```python
from build123d import *

# Parameters (mm, degrees)
SKETCH1_R           = 3.175
BOSS_EXTRUDE1_DEPTH = 2.794
SKETCH2_R           = 11.049
SKETCH2_R_2         = 15.875
SKETCH2_R_3         = 1.27
CUT_EXTRUDE1_DEPTH  = 202.908472752
ITC_CUTOUT_DEPTH    = 202.908472752
SKETCH6_W           = 67.523241089
SKETCH6_H           = 6.35
CUT_EXTRUDE3_DEPTH  = 202.908472752
FILLET1_R           = 6.35
CUT_EXTRUDE4_DEPTH  = 202.908472752
FILLET2_R           = 6.35
SKETCH8_R           = 1.5875
CUT_EXTRUDE5_DEPTH  = 202.908472752
SKETCH10_R          = 1.5875
CUT_EXTRUDE6_DEPTH  = 202.908472752
SKETCH11_R          = 1.5875
CUT_EXTRUDE7_DEPTH  = 202.908472752


with BuildPart() as part:
    # Sketch1 → Boss-Extrude1 (new, symmetric)
    with BuildSketch(Plane.XY):
        with BuildLine():
            Line((-145.783553311, 66.675), (145.783553311, 66.675))
            ThreePointArc((145.783553311, 66.675), (147.900219978, 66.497368874), (149.957676269, 65.969444444))
            ThreePointArc((149.957676269, 65.969444444), (172.789871953, 52.74760778), (189.088888889, 31.999880883))
            ThreePointArc((189.088888889, 31.999880883), (190.142181511, 29.17513943), (190.5, 26.181720723))
            Line((190.5, 26.181720723), (190.5, -22.225))
            ThreePointArc((190.5, -22.225), (186.780256121, -31.205256121), (177.8, -34.925))
            Line((177.8, -34.925), (-177.8, -34.925))
            ThreePointArc((-177.8, -34.925), (-186.780256121, -31.205256121), (-190.5, -22.225))
            Line((-190.5, -22.225), (-190.5, 26.181720723))
            ThreePointArc((-190.5, 26.181720723), (-190.142181511, 29.17513943), (-189.088888889, 31.999880883))
            ThreePointArc((-189.088888889, 31.999880883), (-172.789871953, 52.74760778), (-149.957676269, 65.969444444))
            ThreePointArc((-149.957676269, 65.969444444), (-147.900219978, 66.497368874), (-145.783553311, 66.675))
        make_face()
        with Locations((-127, 0)):
            Circle(SKETCH1_R, mode=Mode.SUBTRACT)
        with Locations((127, 0)):
            Circle(SKETCH1_R, mode=Mode.SUBTRACT)
    extrude(amount=BOSS_EXTRUDE1_DEPTH, both=True)

    # Sketch2 → Cut-Extrude1 (cut, through all)
    with BuildSketch(Plane.XY.offset(2.794)):
        with Locations((-127, 0)):
            Circle(SKETCH2_R)
        with Locations((-160.3375, 0)):
            Circle(SKETCH2_R_2)
        with Locations((-143.499519773, 16.837980227)):
            Circle(SKETCH2_R_3)
        with Locations((-160.3375, 23.8125)):
            Circle(SKETCH2_R_3)
        with Locations((-143.499519773, -16.837980227)):
            Circle(SKETCH2_R_3)
        with Locations((-160.3375, -23.8125)):
            Circle(SKETCH2_R_3)
        with Locations((-177.175480227, -16.837980227)):
            Circle(SKETCH2_R_3)
        with Locations((-184.15, 0)):
            Circle(SKETCH2_R_3)
        with Locations((-177.175480227, 16.837980227)):
            Circle(SKETCH2_R_3)
        with Locations((-127, 15.875)):
            Circle(SKETCH2_R_3)
        with Locations((-115.774679849, 11.225320151)):
            Circle(SKETCH2_R_3)
        with Locations((-111.125, 0)):
            Circle(SKETCH2_R_3)
        with Locations((-115.774679849, -11.225320151)):
            Circle(SKETCH2_R_3)
        with Locations((-127, -15.875)):
            Circle(SKETCH2_R_3)
        with Locations((-138.225320151, -11.225320151)):
            Circle(SKETCH2_R_3)
        with Locations(Location((138.225320151, 11.225320151, 0), (0, 0, 180))):
            Circle(SKETCH2_R_3)
        with Locations((-138.225320151, 11.225320151)):
            Circle(SKETCH2_R_3)
        with Locations(Location((138.225320151, -11.225320151, 0), (0, 0, 180))):
            Circle(SKETCH2_R_3)
        with Locations(Location((127, -15.875, 0), (0, 0, 180))):
            Circle(SKETCH2_R_3)
        with Locations(Location((115.774679849, -11.225320151, 0), (0, 0, 180))):
            Circle(SKETCH2_R_3)
        with Locations(Location((111.125, 0, 0), (0, 0, 180))):
            Circle(SKETCH2_R_3)
        with Locations(Location((115.774679849, 11.225320151, 0), (0, 0, 180))):
            Circle(SKETCH2_R_3)
        with Locations(Location((127, 15.875, 0), (0, 0, 180))):
            Circle(SKETCH2_R_3)
        with Locations(Location((177.175480227, 16.837980227, 0), (0, 0, 180))):
            Circle(SKETCH2_R_3)
        with Locations(Location((184.15, 0, 0), (0, 0, 180))):
            Circle(SKETCH2_R_3)
        with Locations(Location((177.175480227, -16.837980227, 0), (0, 0, 180))):
            Circle(SKETCH2_R_3)
        with Locations(Location((160.3375, -23.8125, 0), (0, 0, 180))):
            Circle(SKETCH2_R_3)
        with Locations(Location((143.499519773, -16.837980227, 0), (0, 0, 180))):
            Circle(SKETCH2_R_3)
        with Locations(Location((160.3375, 23.8125, 0), (0, 0, 180))):
            Circle(SKETCH2_R_3)
        with Locations(Location((143.499519773, 16.837980227, 0), (0, 0, 180))):
            Circle(SKETCH2_R_3)
        with Locations(Location((160.3375, 0, 0), (0, 0, 180))):
            Circle(SKETCH2_R_2)
        with Locations(Location((127, 0, 0), (0, 0, 180))):
            Circle(SKETCH2_R)
    extrude(amount=-CUT_EXTRUDE1_DEPTH, mode=Mode.SUBTRACT)

    # Sketch5 → ITC_Cutout (cut, through all)
    with BuildSketch(Plane.XY.offset(2.794)):
        with BuildLine():
            Line((-88.9, 15.875), (88.9, 15.875))
            ThreePointArc((88.9, 15.875), (97.880256121, 19.594743879), (101.6, 28.575))
            Line((101.6, 28.575), (101.6, 66.675))
            Line((101.6, 66.675), (-101.6, 66.675))
            Line((-101.6, 66.675), (-101.6, 28.575))
            ThreePointArc((-101.6, 28.575), (-97.880256121, 19.594743879), (-88.9, 15.875))
        make_face()
    extrude(amount=-ITC_CUTOUT_DEPTH, mode=Mode.SUBTRACT)

    # Sketch6 → Cut-Extrude3 (cut, through all)
    with BuildSketch(Plane.XY.offset(2.794)):
        with Locations((-105.671932766, 63.5)):
            Rectangle(SKETCH6_W, SKETCH6_H)
        with Locations((105.671932766, 63.5)):
            Rectangle(SKETCH6_W, SKETCH6_H)
    extrude(amount=-CUT_EXTRUDE3_DEPTH, mode=Mode.SUBTRACT)

    # Fillet1
    fillet1_edges = [part.edges().sort_by_distance(p)[0] for p in [
        (-101.6, 60.325, 0),
        (101.6, 60.325, 0),
    ]]
    fillet(fillet1_edges, radius=FILLET1_R)

    # Sketch7 → Cut-Extrude4 (cut, through all)
    with BuildSketch(Plane.XY.offset(2.794)):
        with BuildLine():
            Line((-88.9, -15.875), (88.9, -15.875))
            ThreePointArc((88.9, -15.875), (97.880256121, -19.594743879), (101.6, -28.575))
            Line((101.6, -28.575), (101.6, -34.925))
            Line((101.6, -34.925), (-101.6, -34.925))
            Line((-101.6, -34.925), (-101.6, -28.575))
            ThreePointArc((-101.6, -28.575), (-97.880256121, -19.594743879), (-88.9, -15.875))
        make_face()
    extrude(amount=-CUT_EXTRUDE4_DEPTH, mode=Mode.SUBTRACT)

    # Fillet2
    fillet2_edges = [part.edges().sort_by_distance(p)[0] for p in [
        (101.6, -34.925, 0),
        (-101.6, -34.925, 0),
    ]]
    fillet(fillet2_edges, radius=FILLET2_R - 0.0001)  # a hair under: the kernel refuses the full size

    # Sketch8 → Cut-Extrude5 (cut, through all)
    with BuildSketch(Plane.XY.offset(2.794)):
        with Locations((-135.369553311, 53.975)):
            Circle(SKETCH8_R)
        with Locations((-105.524553311, 53.975)):
            Circle(SKETCH8_R)
        with Locations(Location((105.524553311, 53.975, 0), (0, 0, 180))):
            Circle(SKETCH8_R)
        with Locations(Location((135.369553311, 53.975, 0), (0, 0, 180))):
            Circle(SKETCH8_R)
    extrude(amount=-CUT_EXTRUDE5_DEPTH, mode=Mode.SUBTRACT)

    # Sketch10 → Cut-Extrude6 (cut, through all)
    with BuildSketch(Plane.XY.offset(2.794)):
        with Locations((-177.8, -28.575)):
            Circle(SKETCH10_R)
        with Locations((-107.95, -28.575)):
            Circle(SKETCH10_R)
        with Locations(Location((107.95, -28.575, 0), (0, 0, 180))):
            Circle(SKETCH10_R)
        with Locations(Location((177.8, -28.575, 0), (0, 0, 180))):
            Circle(SKETCH10_R)
        Circle(SKETCH10_R)
    extrude(amount=-CUT_EXTRUDE6_DEPTH, mode=Mode.SUBTRACT)

    # Sketch11 → Cut-Extrude7 (cut, through all)
    with BuildSketch(Plane.XY.offset(2.794)):
        with Locations((-82.55, -9.525)):
            Circle(SKETCH11_R)
        with Locations((-52.705, -9.525)):
            Circle(SKETCH11_R)
        with Locations(Location((52.705, -9.525, 0), (0, 0, 180))):
            Circle(SKETCH11_R)
        with Locations(Location((82.55, -9.525, 0), (0, 0, 180))):
            Circle(SKETCH11_R)
    extrude(amount=-CUT_EXTRUDE7_DEPTH, mode=Mode.SUBTRACT)


solid = part.part
```
Geometry: final body of the model. Coordinates: model frame, mm. A direction names the side the tool comes from. Give positions to 0.01 mm unless a question says otherwise; leave off trailing zeros. Use CSV: the item, a comma, the result in double quotes.
(1) Cut plane A-A (z = -0.05). Count the separate pieces of the cut face and the enclosed holes in it, plus the area to 3 significant figures.
From the geometry:
separate pieces,"1"
enclosed holes,"45"
area,"20,300 mm^2"
(2) Pull-direction query (Y, two-part tool) for faces 1 (the face through (-103.509, -33.114, -0.039)), 2 (the face through (-138.04, 0.49, 0.04)), 3 (the face through (103.51, 58.514, -0.039)); classes: released by +Y, released by -Y, zero draft, split by the parting line, or undercut.
From the geometry:
face 1,"released by -Y"
face 2,"undercut"
face 3,"released by +Y"
(3) Access query for faces 4 (the face through (-97.978, 19.694, 0.039)), 5 (the face through (-97.978, -19.694, 0.039)), 6 (the face through (172.935, 9.66, 0.039)). Directions: +Z, -Z, +X, -X, +Y, -Y. A direction counts if a zero-diameter tool reaches every point of the face in a straight line with its end or side. Return the directions, or none.
From the geometry:
face 4,"+Z, -Z, +Y"
face 5,"+Z, -Z, -Y"
face 6,"+Z, -Z"
(4) First-contact query: P1, Ø3.5, axis at x = 143.5, y = -16.84, coming from the -Z side; P2, Ø3, axis at x = 9, z = -0.5, coming from the +Y side (3 decimals). Flat tips, straight axial feed; report the tip coordinate or a pass-through.
From the geometry:
P1,"z = -2.79"
P2,"y = 15.875"
(5) Ray query, line 1 along X through (y, z) = (27.5, 0.65); line 2 along X through (y, z) = (49.5, -0.45); line 3 along X through (y, z) = (-7, -1.6). Return the intervals inside material, ascending. Write a range as [from, to].
From the geometry:
line 1,"[-190.43, -101.55], [101.55, 190.43]"
line 2,"[-176.28, -101.6], [101.6, 176.28]"
line 3,"[-190.5, -174.59], [-146.09, -135.55], [-118.45, 118.45], [135.55, 146.09], [174.59, 190.5]"
